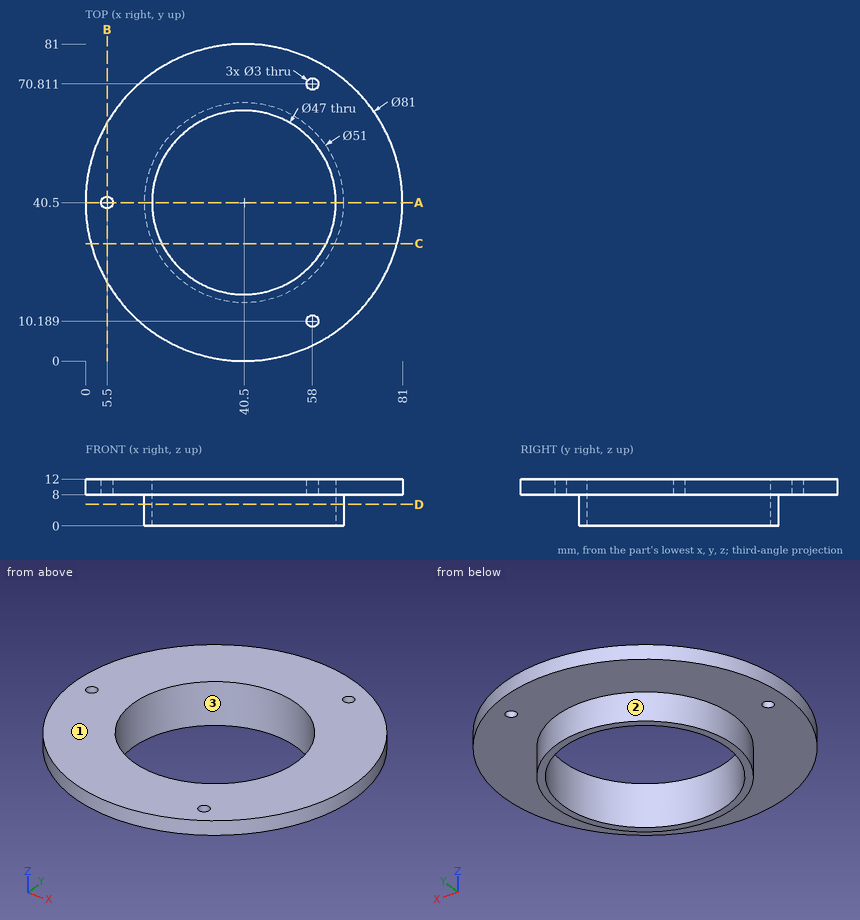
Could you check a few things on this drawing? It's one solid part, dimensions in mm from its lowest x, y, z. Round coordinates to 2 decimals unless told otherwise and drop trailing zeros. Order: outer loops, then holes, each group sorted by start corner. A loop starts at its lowest first (then second) coordinate and runs counter-clockwise, first axis right, second up.
Q1. Please list where these lines run through material, in increasing order: probe 1 along Y at (x, z) = (58, 9.9) (1 decimal); probe 2 along Z at (x, y) = (60, 60); probe 3 along Y at (x, z) = (40.5, 6).
Geometry says:
probe 1: y = 4 to 8.7, 11.7 to 24.8, 56.2 to 69.3, 72.3 to 77
probe 2: z = 8 to 12
probe 3: y = 15 to 17, 64 to 66
Q2. Thinking about a two-plate mould opening in Y: for the marked faces 1, 2 and 3, which applies, released by +Y, released by -Y, zero draft, split by the parting line, or undercut?
Geometry says:
face 1: zero draft
face 2: split by the parting line
face 3: undercut
Q3. I'm going to push flat-ended pins straight in: P1, Ø1, axis at y = 51.5, z = 3.5, coming from the +X side; P2, Ø2, axis at y = 57.5, z = 2.5, coming from the -X side; P3, Ø5, axis at x = 64, z = 9.5, coming from the +Y side. Where does each tip first touch, or does it pass through?
Geometry says:
P1: stops at x = 63.74
P2: stops at x = 20.64
P3: stops at y = 75.13
Q4. Imagine slicing it at B-B, the plane x = 5.5. List the corners of the cut face in (y, z) for me.
Geometry says:
outline: (20.12, 8) - (39, 8) - (39, 12) - (20.12, 12) - close; (42, 8) - (60.88, 8) - (60.88, 12) - (42, 12) - close
Q5. Imagine slicing it at D-D, the plane z = 5.5. List the corners of the cut face in (x, y) for me, then the cut area to 3 significant figures.
Geometry says:
outline: circle Ø51 at (40.5, 40.5); hole circle Ø47 at (40.5, 40.5)
area: 308 mm2
Q6. Imagine slicing it at C-C, the plane y = 30. List the corners of the cut face in (x, z) for me, then the cut area to 3 significant figures.
Geometry says:
outline: (1.38, 8) - (17.26, 8) - (17.26, 0) - (19.48, 0) - (19.48, 12) - (1.38, 12) - close; (61.52, 0) - (63.74, 0) - (63.74, 8) - (79.62, 8) - (79.62, 12) - (61.52, 12) - close
area: 180 mm2
Q7. Imagine slicing it at A-A, the plane y = 40.5. List the corners of the cut face in (x, z) for me, then the cut area to 3 significant figures.
Geometry says:
outline: (0, 8) - (4, 8) - (4, 12) - (0, 12) - close; (7, 8) - (15, 8) - (15, 0) - (17, 0) - (17, 12) - (7, 12) - close; (64, 0) - (66, 0) - (66, 8) - (81, 8) - (81, 12) - (64, 12) - close
area: 156 mm2
